Read the model definition and answer for the solid it produces. Units are mm, in the model's axes. Coordinates: 2 decimals unless noted, no trailing zeros. Order: outer loops, then holes, each group sorted by start corner. A loop starts at its lowest first (then second) coordinate and runs counter-clockwise, first axis right, second up. Notation, with made-up numbers: M -3.75,51.25 L 26.25,51.25 A22 cw 26.25,86.25 Z; hole C 12.25,-0.75 d8. An arc over 180 degrees is marked long. Write each question's results on one line, items separated by ' | '.
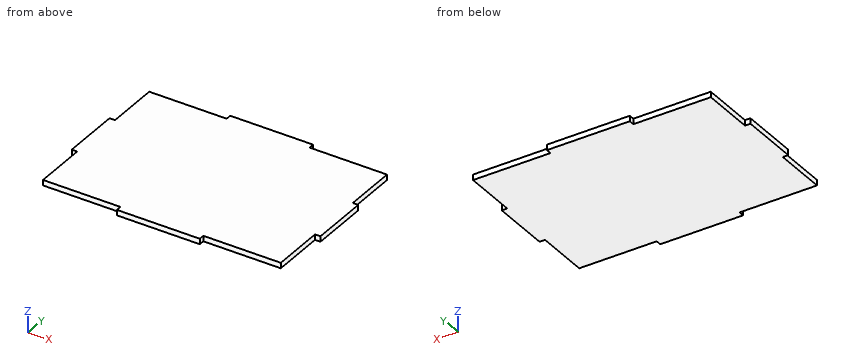
```python
from build123d import *

# Parameters (mm, degrees)
SKETCH1_W           = 231.14
SKETCH1_H           = 162.56
BOSS_EXTRUDE1_DEPTH = 5.08
CAVITY1_START       = -115.57
CAVITY1_OUTLINE_W   = 5.08
CAVITY1_OUTLINE_H   = 5.08
CAVITY1_DEPTH       = 77.046666667
CAVITY1_START_2     = 38.523333333
CAVITY1_2_OUTLINE_W = 5.08
CAVITY1_2_OUTLINE_H = 5.08
CAVITY1_2_DEPTH     = 77.046666667
CAVITY1_3_OUTLINE_W = 49.106666667
CAVITY1_3_OUTLINE_H = 5.08
CAVITY1_3_DEPTH     = 5.08
CAVITY1_START_3     = 110.49
CAVITY1_4_OUTLINE_W = 49.106666667
CAVITY1_4_OUTLINE_H = 5.08
CAVITY1_4_DEPTH     = 5.08


# Read off the part's stored shape, not the designer's step: Cavity1
with BuildPart() as part:
    # Sketch1 → Boss-Extrude1 (new body)
    with BuildSketch(Plane.XY):
        Rectangle(SKETCH1_W, SKETCH1_H)
    extrude(amount=BOSS_EXTRUDE1_DEPTH)

    # Cavity1 outline → Cavity1 (cut)
    with BuildSketch(Plane.YZ.offset(CAVITY1_START)):
        with Locations((78.74, 2.54)):
            Rectangle(CAVITY1_OUTLINE_W, CAVITY1_OUTLINE_H)
        with Locations((-78.74, 2.54)):
            Rectangle(CAVITY1_OUTLINE_W, CAVITY1_OUTLINE_H)
    extrude(amount=CAVITY1_DEPTH, mode=Mode.SUBTRACT)

    # Cavity1 2 outline → Cavity1 2 (cut)
    with BuildSketch(Plane.YZ.offset(CAVITY1_START_2)):
        with Locations((78.74, 2.54)):
            Rectangle(CAVITY1_2_OUTLINE_W, CAVITY1_2_OUTLINE_H)
        with Locations((-78.74, 2.54)):
            Rectangle(CAVITY1_2_OUTLINE_W, CAVITY1_2_OUTLINE_H)
    extrude(amount=CAVITY1_2_DEPTH, mode=Mode.SUBTRACT)

    # Cavity1 3 outline → Cavity1 3 (cut)
    with BuildSketch(Plane.YZ.offset(CAVITY1_START)):
        with Locations((51.646666667, 2.54)):
            Rectangle(CAVITY1_3_OUTLINE_W, CAVITY1_3_OUTLINE_H)
        with Locations((-51.646666667, 2.54)):
            Rectangle(CAVITY1_3_OUTLINE_W, CAVITY1_3_OUTLINE_H)
    extrude(amount=CAVITY1_3_DEPTH, mode=Mode.SUBTRACT)

    # Cavity1 4 outline → Cavity1 4 (cut)
    with BuildSketch(Plane.YZ.offset(CAVITY1_START_3)):
        with Locations((51.646666667, 2.54)):
            Rectangle(CAVITY1_4_OUTLINE_W, CAVITY1_4_OUTLINE_H)
        with Locations((-51.646666667, 2.54)):
            Rectangle(CAVITY1_4_OUTLINE_W, CAVITY1_4_OUTLINE_H)
    extrude(amount=CAVITY1_4_DEPTH, mode=Mode.SUBTRACT)


solid = part.part
```
(1) The part is cut by section C-C, the plane x = 77.5. Write down the section's boundary in (y, z), then the cut area to 3 significant figures.
Conclusion:
outline: M -76.2,0 L 76.2,0 L 76.2,5.08 L -76.2,5.08 Z | area: 774 mm²
(2) Given pin 1 (1 mm diameter, centred on x = -60, z = 2.5, fed in from +Y); pin 2 (1.5 mm diameter, centred on y = 63.5, z = 2.5, fed in from -X); pin 3 (2.5 mm diameter, centred on x = -113, z = 2, fed in from +Y), each flat-ended and moving along its own axis, determine where each tip first touches the part or whether it passes through.
Conclusion:
pin 1: y = 76.2 | pin 2: x = -110.49 | pin 3: y = 27.09
(3) Straight lines are drawn through the part: line 1 (X direction, y = 46, z = 1.95); line 2 (Y direction, x = 103, z = 0.3). For each, find the intervals that lie inside material, in ascending order.
Conclusion:
line 1: -110.49 to 110.49 | line 2: -76.2 to 76.2
(4) The part is cut by section A-A, the plane z = 3.25. Write down the section's boundary in (x, y).
Conclusion:
outline: M -115.57,-27.09 L -110.49,-27.09 L -110.49,-76.2 L -38.52,-76.2 L -38.52,-81.28 L 38.52,-81.28 L 38.52,-76.2 L 110.49,-76.2 L 110.49,-27.09 L 115.57,-27.09 L 115.57,27.09 L 110.49,27.09 L 110.49,76.2 L 38.52,76.2 L 38.52,81.28 L -38.52,81.28 L -38.52,76.2 L -110.49,76.2 L -110.49,27.09 L -115.57,27.09 Z
(5) The part is cut by section B-B, the plane y = -44. Write down the section's boundary in (x, z).
Conclusion:
outline: M -110.49,0 L 110.49,0 L 110.49,5.08 L -110.49,5.08 Z
